Input: part model. Units: mm. Frame: model coordinates. A direction names the side the tool comes from. Round coordinates to 2 decimals unless told otherwise and drop trailing zeros. Order: outer loops, then holes, each group sorted by start corner. A loop starts at its lowest first (then second) coordinate and runs counter-clockwise, first axis right, second up. Notation, with made-up numbers: (86.5, 87) - (96.5, 87) arc R18 ccw to (96.5, 91) - close; hole circle Ø5 at (36.25, 21). An arc over 180 degrees is marked (long way). One line per item, written item: value. Start each with the question number.
from build123d import *

# Parameters (mm, degrees)
SKETCH2_W           = 81
SKETCH2_H           = 53
BOSS_EXTRUDE1_DEPTH = 10
BOSS_EXTRUDE2_DEPTH = 10
BOSS_EXTRUDE3_DEPTH = 10


with BuildPart() as part:
    # Sketch2 → Boss-Extrude1 (new body)
    with BuildSketch(Plane(origin=(0, 0, 0), x_dir=(1, 0, 0), z_dir=(0, 1, 0))):
        Polygon((77.422904192, 25), (77.422904192, 53), (42.44011976, 53), (42.44011976, 0), align=None)
        with Locations((1.94011976, 26.5)):
            Rectangle(SKETCH2_W, SKETCH2_H)
    extrude(amount=-BOSS_EXTRUDE1_DEPTH)

    # Sketch3 → Boss-Extrude2 (add)
    with BuildSketch(Plane(origin=(0, 0, -53), x_dir=(-1, 0, 0), z_dir=(0, 0, -1))):
        Polygon((-77.422904192, 0), (-77.422904192, 39.932268243), (-9.422904192, 39.932268243), (28.55988024, 0), align=None)
    extrude(amount=-BOSS_EXTRUDE2_DEPTH)

    # Sketch4 → Boss-Extrude3 (add)
    with BuildSketch(Plane(origin=(32.422904192, 0, 0), x_dir=(0, 0, -1), z_dir=(1, 0, 0))):
        Polygon((43, 39.932268243), (5, 0), (43, 0), align=None)
    extrude(amount=-BOSS_EXTRUDE3_DEPTH)


solid = part.part
1. Line query: line 1 (Y direction, x = 20, z = -42); line 2 (Z direction, x = 45, y = 24); line 3 (X direction, y = 25, z = -38.5). Output: solid intervals per line, ascending. Write a range as from..to.
2. Set-up query: faces 1 (the face through (2, 16, -43)), 2 (the face through (6, 0, -21)), 3 (the face through (-9.3, 20.25, -48.07)), 4 (the face through (55, 20, -43)). Return all of +Z, -Z, +X, -X, +Y, -Y with unobstructed straight access to the full face (end or side cutting, diameter ignored); none if empty.
3. Section B-B (z = -47.5). Return the cut outline in (x, y).
4. Pin query (flat end, axial travel): pin 1 (19 mm diameter, centred on y = 11.5, z = -23, fed in from +X); pin 2 (10 mm diameter, centred on x = 54.5, z = -29, fed in from +Y); pin 3 (12 mm diameter, centred on x = 8, y = 11, fed in from +Z). Return the tip coordinate at first contact, or that it passes through.
5. Section D-D (z = -22). Return the cut outline in (x, y), then the cut area to 3 significant figures.
6. Section C-C (y = 15). Return the cut outline in (x, z).
7. Section A-A (x = 34.5). Return the cut outline in (y, z).
Solved:
1. line 1: y = -10..0
1. line 2: z = -53..-43
1. line 3: x = 22.42..32.42
2. face 1: +Z, -X, +Y
2. face 2: +Z, +Y
2. face 3: +Z, -Z, -X, +Y
2. face 4: +Z, +X, +Y
3. outline: (-38.56, -10) - (77.42, -10) - (77.42, 39.93) - (9.42, 39.93) - (-28.56, 0) - (-38.56, 0) - close
4. pin 1: stops at x = 32.42
4. pin 2: stops at y = 0
4. pin 3: stops at z = -43
5. outline: (-38.56, -10) - (73.22, -10) - (73.22, 0) - (32.42, 0) - (32.42, 17.86) - (22.42, 17.86) - (22.42, 0) - (-38.56, 0) - close
5. area: 1,300 mm²
6. outline: (-14.29, -53) - (77.42, -53) - (77.42, -43) - (32.42, -43) - (32.42, -19.27) - (22.42, -19.27) - (22.42, -43) - (-14.29, -43) - close
7. outline: (-10, -53) - (39.93, -53) - (39.93, -43) - (0, -43) - (0, 0) - (-10, 0) - close
